```python
from build123d import *

# Parameters (mm, degrees)
F1_DEPTH = 25.4
F2_DEPTH = 25.4
F3_DEPTH = 25.4
F4_DEPTH = 25.4
F5_DEPTH = 25.4


with BuildPart() as f1:
    # F0 (on Top) → F1 (new body)
    with BuildSketch(Plane.XY):
        Polygon((29.9969874322, 40.0068945546), (29.9969874322, 6.1151932525), (51.8570691347, 5.7021006942), align=None)
        Polygon((51.8570691347, 5.7021006942), (29.9969874322, 6.1151932525), (29.9969874322, -50.8127212524), (68.4659332037, 42.1804785728), (29.9969874322, 42.1804785728), (29.9969874322, 40.0068945546), align=None)
        Polygon((-0.1684613526, 87.345212698), (29.9969874322, 40.0068945546), (29.9969874322, 42.1804785728), (29.9969874322, 135.1736783981), align=None)
    extrude(amount=F1_DEPTH)

    # F2 (add): a face of the model
    f2_faces = [f1.faces().sort_by_distance(p)[0] for p in [
        (29.9969874322, 88.6770784855, 12.7),
    ]]
    extrude(f2_faces, amount=F2_DEPTH)

    # F3 (add): a face of the model
    f3_faces = [f1.faces().sort_by_distance(p)[0] for p in [
        (36.8893007779, 63.5629589231, 0),
    ]]
    extrude(f3_faces, amount=F3_DEPTH)

    # F4 (add): a face of the model
    f4_faces = [f1.faces().sort_by_distance(p)[0] for p in [
        (61.931460318, 42.1804785728, 0),
    ]]
    extrude(f4_faces, amount=F4_DEPTH)

    # F5 (add): a face of the model
    f5_faces = [f1.faces().sort_by_distance(p)[0] for p in [
        (29.9969874322, -5.4029133489, 0),
    ]]
    extrude(f5_faces, amount=F5_DEPTH)


solid = f1.part
```
Geometry check sheet. Reference: the model listing, model coordinates, mm. A direction names the side the tool comes from. Coordinates: 2 decimals unless noted, no trailing zeros. Loops run counter-clockwise (first coordinate to the right, second up) from the corner with the lowest first, then second, coordinate; pieces in that order, holes last.
Item 1: Thickness scan on line 1 (Y direction, x = 13.5, z = 6); line 2 (Y direction, x = 23, z = 13); line 3 (X direction, y = 4, z = -5.5). Record the ranges inside material, lowest first.
Item 2: Sectioned sample at B-B, the plane x = 39. Record the boundary of the cut face in (y, z).
Item 3: Go/stop test with flat-tipped pins: pin 1 Ø4 at (y, z) = (115.5, -4) entering from -X; pin 2 Ø6.5 at (x, z) = (60, -12.5) entering from +Y; pin 3 Ø20.5 at (x, z) = (18.5, 8.5) entering from +Y. Record where each tip stops, or that it passes through.
Item 4: Sectioned sample at C-C, the plane y = -5. Record the boundary of the cut face in (x, z), then the cut area to 3 significant figures.
Item 5: Release check for a two-part mould opening along Y. For faces 1 (the face through (35, 43, 25.4)), 2 (the face through (17, -50.813, 0)), 3 (the face through (14.7, 64.01, 0.36)) record: released by +Y, released by -Y, zero draft, split by the parting line, or undercut.
Item 6: Access from +Z, -Z, +X, -X, +Y, -Y to the whole of each face (thin tool, end or side, straight path). Record for faces 4 (the face through (4.597, -5, 0)), 5 (the face through (15.125, 111.594, 0.356)), 6 (the face through (55.397, 101, 0)), 7 (the face through (17, 40.007, 0)).
Item 7: Sectioned sample at A-A, the plane z = 8.5. Record the boundary of the cut face in (x, y), then the cut area to 3 significant figures.
Check result:
1. line 1: y = -50.81 to 40.01, 65.9 to 109.02
1. line 2: y = -50.81 to 40.01, 50.99 to 124.08
1. line 3: x = 4.6 to 52.67
2. outline: (-29.05, -25.4) - (135.17, -25.4) - (135.17, 25.4) - (-29.05, 25.4) - close
3. pin 1: stops at x = 16.33
3. pin 2: stops at y = 67.58
3. pin 3: stops at y = 133.2
4. outline: (4.6, -25.4) - (48.95, -25.4) - (48.95, 25.4) - (4.6, 25.4) - close
4. area: 2,250 mm2
5. face 1: zero draft
5. face 2: released by -Y
5. face 3: undercut
6. face 4: +Z, -Z, -X, -Y
6. face 5: +Z, -Z, -X, +Y
6. face 6: +Z, -Z, +X, +Y
6. face 7: +Z, -Z, -X
7. outline: (-0.17, 87.35) - (30, 40.01) - (4.6, 40.01) - (4.6, -50.81) - (30, -50.81) - (68.47, 42.18) - (68.47, 67.58) - (55.4, 67.58) - (55.4, 135.17) - (30, 135.17) - close
7. area: 8,220 mm2
